Could you check a few things on this drawing? It's one solid part, dimensions in mm from its lowest x, y, z. Coordinates: 2 decimals unless noted, no trailing zeros. Order: outer loops, then holes, each group sorted by start corner. A loop starts at its lowest first (then second) coordinate and runs counter-clockwise, first axis right, second up. Notation, with made-up numbers: (12, 71.25) - (43, 71.25) arc R11 cw to (43, 86.25) - close; hole circle Ø11 at (4.25, 65.5). An arc over 180 degrees is marked (long way). Return JSON: item names as keys, results as strings. Group by question number.
1) If we mould it in two halves opening along Y, with no side actions, what happens to the marked faces 1 and 2? For each: pulls with the +Y half, pulls with the -Y half, needs draft (parallel to the pull), parting line crosses it, or undercut.
2) Imagine slicing it at C-C (x = 93). Write out the boundary of the cut face in (y, z).
3) For pin 1 Ø0.5 at (y, z) = (2, 3.5) entering from -X; pin 2 Ø2 at (x, y) = (13.5, 49) entering from +Z; pin 3 Ø1.7 at (y, z) = (29.5, 3) entering from +X, each with a flat end and sliding along its axis, tell me the tip position at first contact or that it passes through.
4) Imagine slicing it at A-A (z = 3.1). Write out the boundary of the cut face in (x, y).
5) Imagine slicing it at D-D (x = 47.5). Write out the boundary of the cut face in (y, z).
6) If I drill on line 1 along Y through (x, z) = (32, 2.85); line 2 along X through (y, z) = (27, 4.25); line 3 along Z through (x, y) = (71.5, 25.5), over which ranges is the centre line in solid material (lowest first)?
7) Imagine slicing it at B-B (y = 27.5). Write out the boundary of the cut face in (x, z), and give its area (3 significant figures).
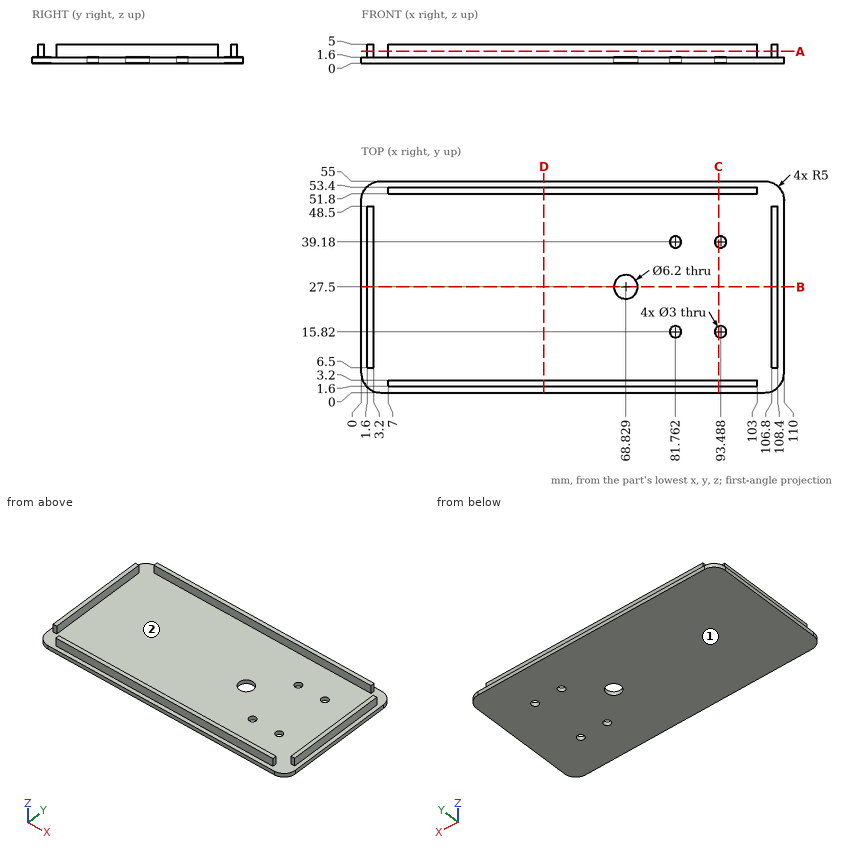
Calculated:
{
 "1": {"face 1": "needs draft", "face 2": "undercut"},
 "2": {"outline": "(0, 0) - (14.4, 0) - (14.4, 1.6) - (3.2, 1.6) - (3.2, 5) - (1.6, 5) - (1.6, 1.6) - (0, 1.6) - close; (17.24, 0) - (37.76, 0) - (37.76, 1.6) - (17.24, 1.6) - close; (40.6, 0) - (55, 0) - (55, 1.6) - (53.4, 1.6) - (53.4, 5) - (51.8, 5) - (51.8, 1.6) - (40.6, 1.6) - close"},
 "3": {"pin 1": "x = 7", "pin 2": "z = 1.6", "pin 3": "x = 108.4"},
 "4": {"outline": "(1.6, 6.5) - (3.2, 6.5) - (3.2, 48.5) - (1.6, 48.5) - close; (7, 1.6) - (103, 1.6) - (103, 3.2) - (7, 3.2) - close; (7, 51.8) - (103, 51.8) - (103, 53.4) - (7, 53.4) - close; (106.8, 6.5) - (108.4, 6.5) - (108.4, 48.5) - (106.8, 48.5) - close"},
 "5": {"outline": "(0, 0) - (55, 0) - (55, 1.6) - (53.4, 1.6) - (53.4, 5) - (51.8, 5) - (51.8, 1.6) - (3.2, 1.6) - (3.2, 5) - (1.6, 5) - (1.6, 1.6) - (0, 1.6) - close"},
 "6": {"line 1": "1.6 to 3.2, 51.8 to 53.4", "line 2": "1.6 to 3.2, 106.8 to 108.4", "line 3": "0 to 1.6"},
 "7": {"outline": "(0, 0) - (65.73, 0) - (65.73, 1.6) - (3.2, 1.6) - (3.2, 5) - (1.6, 5) - (1.6, 1.6) - (0, 1.6) - close; (71.93, 0) - (110, 0) - (110, 1.6) - (108.4, 1.6) - (108.4, 5) - (106.8, 5) - (106.8, 1.6) - (71.93, 1.6) - close", "area": "177 mm2"}
}
